The model under review builds one solid part; all positions refer to its coordinate system, in mm. A direction names the side the tool comes from. Coordinates: 2 decimals unless noted, no trailing zeros. Write each loop counter-clockwise with the first axis right and the second up, starting at its lowest first coordinate (ties: lowest second). Pieces come first, ordered by that corner, then holes. Notation, with made-up numbers: M 17.25,29 L 27.25,29 A13 cw 27.25,44 Z; hole C 55,-35 d7. An arc over 180 degrees is marked long. Answer as a JSON object with one key per item and string values.
Autodesk Fusion 360 part; units mm, degrees
sketch "Sketch2" plane through (0, 0, 0) normal (0, 0, 1) x (1, 0, 0)
  line L0 (0, 0) -> (60, 0)
  line L1 (60, 0) -> (60, 80)
  line L2 (60, 80) -> (0, 80)
  line L3 (0, 80) -> (0, 0)
  line L4 (56, 0) -> (56, 76)
  line L5 (56, 76) -> (4, 76)
  line L6 (4, 76) -> (4, 0)
  line L7 (15, 65) -> (15, 65)
  line L8 (17.5, 62.5) -> (17.5, 17.5)
  line L9 (15, 15) -> (15, 15)
  line L10 (12.5, 17.5) -> (12.5, 62.5)
  line L11 (45, 65) -> (45, 65)
  line L12 (47.5, 62.5) -> (47.5, 17.5)
  line L13 (45, 15) -> (45, 15)
  line L14 (42.5, 17.5) -> (42.5, 62.5)
  arc A0 (15, 65) -> (12.5, 62.5) centre (15, 62.5) ccw
  arc A1 (17.5, 62.5) -> (15, 65) centre (15, 62.5) ccw
  arc A2 (45, 65) -> (42.5, 62.5) centre (45, 62.5) ccw
  arc A3 (47.5, 62.5) -> (45, 65) centre (45, 62.5) ccw
  arc A4 (12.5, 17.5) -> (15, 15) centre (15, 17.5) ccw
  arc A5 (15, 15) -> (17.5, 17.5) centre (15, 17.5) ccw
  arc A6 (42.5, 17.5) -> (45, 15) centre (45, 17.5) ccw
  arc A7 (45, 15) -> (47.5, 17.5) centre (45, 17.5) ccw
  dimension "d1" = 60
  dimension "d2" = 80
  dimension "d3" = 4
  dimension "d4" = 4
  dimension "d5" = 4
  dimension "d7" = 25
  dimension "d8" = 8.5
  dimension "d9" = 5
  dimension "d10" = 5
  dimension "d14" = 2.5
  dimension "d15" = 2.5
  dimension "d16" = 2.5
  dimension "d17" = 2.5
  dimension "d18" = 2.5
  dimension "d19" = 2.5
  dimension "d20" = 15
extrude "Extrude1" add sketch "Sketch2" along normal blind 4 contours L0 L1 L2 L3 L4 L5 L6 | L0 L4 L5 L6 | L8 L10 A0 A1 A4 A5 | L12 L14 A2 A3 A6 A7
extrude "Extrude2" add sketch "Sketch2" along normal blind 80 contours L0 L1 L2 L3 L4 L5 L6
sketch "Sketch3" plane through (60, 0, 0) normal (1, 0, 0) x (0, 1, 0)
  line L0 (0, 0) -> (80, 0)
  line L1 (80, 0) -> (80, 80)
  line L2 (80, 80) -> (0, 80)
  line L3 (0, 80) -> (0, 0)
  line L4 (0, 10) -> (70, 80)
  dimension "d25" = 10
  dimension "d26" = 10
extrude "Extrude3" cut sketch "Sketch3" against normal blind 95 contours L2 L3 L4
extrude "Extrude4" cut sketch "Sketch2" along normal blind 10 contours L8 L10 A0 A1 A4 A5 | L12 L14 A2 A3 A6 A7
(1) For faces 1 (the face through (4, 47, 33)), 2 (the face through (30, 77, 80)), 3 (the face through (12.5, 40, 2)), list the 3-axis set-ups (+Z, -Z, +X, -X, +Y, -Y) from which the entire face can be reached by the end or side of a thin tool; tool diameter is ignored.
Results list:
{"face 1": "+Z, -Y", "face 2": "+Z, +X, -X, +Y, -Y", "face 3": "+Z, -Z"}
(2) Wall thickness on line 1 along X through (y, z) = (11, 12.5); line 2 along Z through (x, y) = (36.5, 34); line 3 along Y through (x, z) = (41.5, 12.5): over which ranges is each line inside the solid? List them lowest first. Write a range as from..to.
Results list:
{"line 1": "0..4, 56..60", "line 2": "0..4", "line 3": "76..80"}
(3) For pin 1 Ø1.5 at (x, y) = (11.5, 65.5) entering from +Z; pin 2 Ø15.5 at (x, z) = (30, 56) entering from -Y; pin 3 Ø8 at (x, z) = (54, 33) entering from -Y, all flat-tipped, find the tip position at first contact; note any pin that passes through.
Results list:
{"pin 1": "z = 4", "pin 2": "y = 76", "pin 3": "y = 19.54"}
(4) Add section B-B on y = 29. Give the boundary of the cut face in (x, z).
Results list:
{"outline": "M 0,0 L 12.5,0 L 12.5,4 L 4,4 L 4,39 L 0,39 Z; M 17.5,0 L 42.5,0 L 42.5,4 L 17.5,4 Z; M 47.5,0 L 60,0 L 60,39 L 56,39 L 56,4 L 47.5,4 Z"}
(5) Add section D-D on y = 12.5. Give the boundary of the cut face in (x, z), and give its area (3 significant figures).
Results list:
{"outline": "M 0,0 L 60,0 L 60,22.5 L 56,22.5 L 56,4 L 4,4 L 4,22.5 L 0,22.5 Z", "area": "388 mm²"}
(6) Add section A-A on x = 45. Give the boundary of the cut face in (y, z), and give its area (3 significant figures).
Results list:
{"outline": "M 0,0 L 15,0 L 15,4 L 0,4 Z; M 65,0 L 80,0 L 80,80 L 76,80 L 76,4 L 65,4 Z", "area": "424 mm²"}
(7) Draft analysis for pull direction Y (two halves, no side actions). For faces 4 (the face through (30, 80, 39)), 5 (the face through (0, 49, 31)), 6 (the face through (30, 76, 41)), 7 (the face through (15, 15, 2)), state which applies: released by +Y, released by -Y, zero draft, split by the parting line, or undercut.
Results list:
{"face 4": "released by +Y", "face 5": "zero draft", "face 6": "released by -Y", "face 7": "undercut"}
(8) Add section C-C on z = 61.5. Give the boundary of the cut face in (x, y).
Results list:
{"outline": "M 0,51.5 L 4,51.5 L 4,76 L 56,76 L 56,51.5 L 60,51.5 L 60,80 L 0,80 Z"}
